Here's how the part is built. I have some questions about the finished solid (model axes, mm). Face numbers are marked on the shaded views. Round coordinates to 2 decimals unless told otherwise and drop trailing zeros. Loops run counter-clockwise (first coordinate to the right, second up) from the corner with the lowest first, then second, coordinate; pieces in that order, holes last. Notation, with made-up numbers: (15, -10.5) - (52, -10.5) arc R15 cw to (52, 6.5) - close; hole circle Ø11 at (42.5, 32.25). An arc over 180 degrees is marked (long way). Return JSON: item names as keys, results as strings. Group by question number.
Autodesk Inventor part; units mm, degrees
ref_plane "YZ Plane" through (0, 0, 0) normal (1, 0, 0) x (0, 1, 0)
ref_plane "XZ Plane" through (0, 0, 0) normal (0, 1, 0) x (-1, 0, 0)
ref_plane "XY Plane" through (0, 0, 0) normal (0, 0, 1) x (1, 0, 0)
sketch "スケッチ1" plane through (0, 0, 0) normal (0, 0, 1) x (1, 0, 0)
  circle A0 centre (0, 0) radius 4.1
  dimension "d0" = 8.2
extrude "押し出し1" add sketch "スケッチ1" along normal blind 10
sketch "スケッチ2" plane through (0, 0, 10) normal (0, 0, 1) x (1, 0, 0)
  circle A0 centre (0, 0) radius 3.5
  dimension "d3" = 7
extrude "押し出し2" add sketch "スケッチ2" along normal blind 5
sketch "スケッチ3" plane through (0, 0, 15) normal (0, 0, 1) x (1, 0, 0)
  circle A0 centre (0, 0) radius 4.1
  circle A1 centre (0, 0) radius 4.1
  circle A2 centre (0, 0) radius 4.1
  point P0 (0, 4.1)
extrude "押し出し3" add sketch "スケッチ3" along normal blind 3
chamfer "面取り1" distance 0.6 angle 45 2 edges at (-3.5, 0, 10) (-3.5, 0, 15)
chamfer "面取り2" distance 0.7 angle 45 2 edges at (-4.1, 0, 18) (-4.1, 0, 0)
fillet "フィレット1" radius 1 2 edges at (-3.5, 0, 10.5995) (-3.5, 0, 14.4005)
properties part number "stopper_inhibitory"
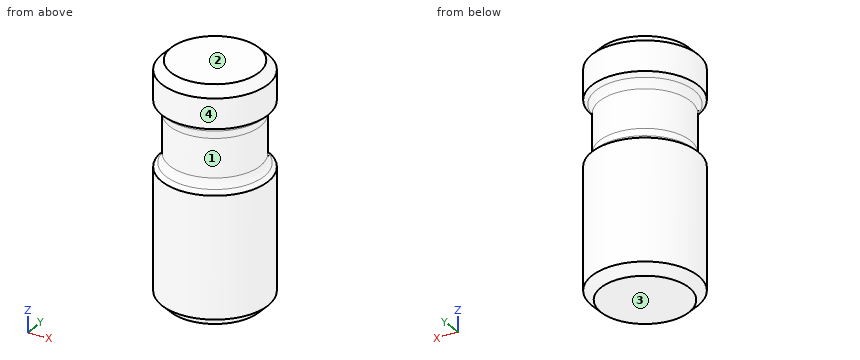
Q1. Imagine slicing it at A-A, the plane z = 13.75. List the corners of the cut face in (x, y) for me.
Q2. Will these pins go through, and if not, where does the flat tip stop? pin 1 Ø1 at (x, z) = (2.5, 12) entering from +Y; pin 2 Ø4 at (x, y) = (3, -2) entering from -Z; pin 3 Ø1 at (x, z) = (1.5, 14.5) entering from -Y; pin 4 Ø2 at (y, z) = (2.5, 12) entering from +X.
Q3. Please list where these lines run through material, in increasing order: line 1 (Z direction, x = -3.5, y = -2); line 2 (X direction, y = -0.5, z = 14.25); line 3 (Z direction, x = -3.5, y = -1.75).
Q4. Imagine slicing it at B-B, the plane z = 6. List the corners of the cut face in (x, y) for me.
Q5. If we mould it in two halves opening along Z, with no side actions, what happens to the marked faces 1, 2, 3 and 4? For each: +Z half, -Z half, draft (parallel to the pull), parting line (faces both ways), or undercut.
Output values:
{
 "1": {"outline": "circle Ø7 at (0, 0)"},
 "2": {"pin 1": "stops at y = 2.87", "pin 2": "stops at z = 0", "pin 3": "stops at y = -3.85", "pin 4": "stops at x = 3.16"},
 "3": {"line 1": "z = 0.63 to 10.07, 14.93 to 17.37", "line 2": "x = -3.5 to 3.5", "line 3": "z = 0.51 to 10.19, 14.81 to 17.49"},
 "4": {"outline": "circle Ø8.2 at (0, 0)"},
 "5": {"face 1": "undercut", "face 2": "+Z half", "face 3": "-Z half", "face 4": "draft"}
}
